from build123d import *

# Parameters (mm, degrees)
ESQUISSE1_R        = 10
ESQUISSE1_R_2      = 2.1
BOSS_EXTRU_1_DEPTH = 3
BOSS_EXTRU_2_DEPTH = 5
BOSS_EXTRU_3_START = 2.45
BOSS_EXTRU_3_DEPTH = 2.45
ESQUISSE4_R        = 10
ESQUISSE4_R_2      = 8
BOSS_EXTRU_4_DEPTH = 2
CONG_5_R           = 2
CONG_6_R           = 2
CONG_7_R           = 2
CONG_8_R           = 2
CONG_10_R          = 0.5
CHANFREIN1_SIZE    = 0.2


with BuildPart() as part:
    # Esquisse1 → Boss.-Extru.1 (new body)
    with BuildSketch(Plane(origin=(0, 0, 0), x_dir=(1, 0, 0), z_dir=(0, 1, 0))):
        with Locations(Location((0, 0, 0), (0, 0, 270))):
            Circle(ESQUISSE1_R)
        with Locations(Location((0, 0, 0), (0, 0, 270))):
            Circle(ESQUISSE1_R_2, mode=Mode.SUBTRACT)
    extrude(amount=BOSS_EXTRU_1_DEPTH)

    # Esquisse2 → Boss.-Extru.2 (add)
    with BuildSketch(Plane(origin=(0, 0, 0), x_dir=(1, 0, 0), z_dir=(0, 1, 0))):
        with BuildLine():
            Line((-9.901515036, -1.4), (-16, -1.4))
            ThreePointArc((-16, -1.4), (-17.4, 0), (-16, 1.4))
            Line((-16, 1.4), (-9.901515036, 1.4))
            ThreePointArc((-9.901515036, 1.4), (-8.501515036, 0), (-9.901515036, -1.4))
        make_face()
        with BuildLine():
            Line((9.901515036, -1.4), (16, -1.4))
            ThreePointArc((16, -1.4), (17.4, 0), (16, 1.4))
            Line((16, 1.4), (9.901515036, 1.4))
            ThreePointArc((9.901515036, 1.4), (8.501515036, 0), (9.901515036, -1.4))
        make_face()
    extrude(amount=BOSS_EXTRU_2_DEPTH)

    # Esquisse3 → Boss.-Extru.3 (add)
    with BuildSketch(Plane.XZ.offset(BOSS_EXTRU_3_START)):
        with BuildLine():
            Line((-10.05, -1.4), (-16, -1.4))
            ThreePointArc((-16, -1.4), (-17.4, 0), (-16, 1.4))
            Line((-16, 1.4), (-10.05, 1.4))
            ThreePointArc((-10.05, 1.4), (-8.65, 0), (-10.05, -1.4))
        make_face()
        with BuildLine():
            Line((10.05, -1.4), (16, -1.4))
            ThreePointArc((16, -1.4), (17.4, 0), (16, 1.4))
            Line((16, 1.4), (10.05, 1.4))
            ThreePointArc((10.05, 1.4), (8.65, 0), (10.05, -1.4))
        make_face()
    extrude(amount=-BOSS_EXTRU_3_DEPTH)

    # Esquisse4 → Boss.-Extru.4 (add)
    with BuildSketch(Plane(origin=(0, 3, 0), x_dir=(1, 0, 0), z_dir=(0, 1, 0))):
        Circle(ESQUISSE4_R)
        with Locations(Location((0, 0, 0), (0, 0, 270))):
            Circle(ESQUISSE4_R_2, mode=Mode.SUBTRACT)
    extrude(amount=BOSS_EXTRU_4_DEPTH)

    # Congé5
    # the kernel refuses this fillet: 2 mm, written as the material it adds along each edge
    with BuildSketch(Plane(origin=(9.901515036, 5, -1.4), x_dir=(1, 0, 0), z_dir=(0, -1, 0))) as cong_5_piece_1:
        with BuildLine():
            CenterArc((1.606742869, -2), CONG_5_R, 90, 73.540750372)
            ThreePointArc((-0.311300115, -1.433333333), (-0.129335377, -0.72238185), (0, 0))
            Line((0, 0), (1.606742869, 0))
        make_face()
    extrude(amount=5)

    # Congé6
    # the kernel refuses this fillet: 2 mm, written as the material it adds along each edge
    with BuildSketch(Plane(origin=(9.901515036, 0, 1.4), x_dir=(1, 0, 0), z_dir=(0, 1, 0))) as cong_6_piece_1:
        with BuildLine():
            CenterArc((1.606742869, -2), CONG_6_R, 90, 73.540750372)
            ThreePointArc((-0.311300115, -1.433333333), (-0.129335377, -0.72238185), (0, 0))
            Line((0, 0), (1.606742869, 0))
        make_face()
    extrude(amount=5)

    # Congé7
    # the kernel refuses this fillet: 2 mm, written as the material it adds along each edge
    with BuildSketch(Plane(origin=(-9.901515036, 5, -1.4), x_dir=(0.2122381850229741, 0, -0.9772179658695156), z_dir=(0, -1, 0))) as cong_7_piece_1:
        with BuildLine():
            CenterArc((1.613423741, -1.994614368), CONG_7_R, 94.20570169, 73.540750372)
            Line((-0.34101219, -1.570137998), (0, 0))
            ThreePointArc((0, 0), (0.733374428, -0.026928159), (1.466748856, 0))
        make_face()
    extrude(amount=5)

    # Congé8
    # the kernel refuses this fillet: 2 mm, written as the material it adds along each edge
    with BuildSketch(Plane(origin=(-9.901515036, 5, 1.4), x_dir=(0.21223818502297503, 0, 0.9772179658695155), z_dir=(0, -1, 0))) as cong_8_piece_1:
        with BuildLine():
            CenterArc((1.613423741, 1.994614368), CONG_8_R, 192.253547938, 73.540750372)
            Line((-0.34101219, 1.570137998), (0, 0))
            ThreePointArc((0, 0), (0.733374428, 0.026928159), (1.466748856, 0))
        make_face()
    extrude(amount=5)

    # Congé10
    cong_10_edges = [part.edges().sort_by_distance(p)[0] for p in [
        (-8.65, -2.45, 0),
        (-13.025, -2.45, 1.4),
        (-17.4, -2.45, 0),
        (-13.025, -2.45, -1.4),
        (8.65, -2.45, 0),
        (13.025, -2.45, -1.4),
        (17.4, -2.45, 0),
        (13.025, -2.45, 1.4),
    ]]
    fillet(cong_10_edges, radius=CONG_10_R)

    # Chanfrein1
    chanfrein1_edges = [part.edges().sort_by_distance(p)[0] for p in [
        (0, 5, -8),
    ]]
    chamfer(chanfrein1_edges, length=CHANFREIN1_SIZE)


solid = part.part
Geometry check sheet. Reference: the model listing, model coordinates, mm. A direction names the side the tool comes from. Give positions to 0.01 mm unless a question says otherwise; leave off trailing zeros. Order: outer loops, then holes, each group sorted by start corner. A loop starts at its lowest first (then second) coordinate and runs counter-clockwise, first axis right, second up.
1) Draft check along Z on faces 4 (the cylindrical face through (-7.81, 3.89, -1.73)), 5 (the cylindrical face through (-10.325, 2.535, 1.787)), 6 (the cylindrical face through (0, 2, -10)). Enter one of: released by +Z, released by -Z, zero draft, split by the parting line, or undercut.
Results are:
face 4: undercut
face 5: released by +Z
face 6: released by -Z
2) Tool access check on faces 1 (the flat face through (-2, 3, 2)), 2 (the cylindrical face through (17.4, 1.5, 0)), 3 (the cylindrical face through (8.65, -0.99, 0.03)). Record the directions out of +Z, -Z, +X, -X, +Y, -Y that give a thin tool (end or side, any length) a straight path to the whole face; none if there is none.
Results are:
face 1: +Y
face 2: +X, +Y, -Y
face 3: -Y
3) Cross-section at B-B (y = -0.5). Record the boundary of the cut face in (x, z), then the cut area to 3 significant figures.
Results are:
outline: (-16, -1.4) - (-10.05, -1.4) arc R1.4 ccw to (-10.05, 1.4) - (-16, 1.4) arc R1.4 ccw to start; (10.05, -1.4) - (16, -1.4) arc R1.4 ccw to (16, 1.4) - (10.05, 1.4) arc R1.4 ccw to start
area: 45.6 mm2
4) Cross-section at C-C (y = 2.5). Record the boundary of the cut face in (x, z).
Results are:
outline: (-16, -1.4) - (-11.51, -1.4) arc R2 cw to (-9.59, -2.83) arc R10 ccw to (9.59, -2.83) arc R2 cw to (11.51, -1.4) - (16, -1.4) arc R1.4 ccw to (16, 1.4) - (11.51, 1.4) arc R2 cw to (9.59, 2.83) arc R10 ccw to (-9.59, 2.83) arc R2 cw to (-11.51, 1.4) - (-16, 1.4) arc R1.4 ccw to start; hole circle Ø4.2 at (0, 0)
5) Cross-section at D-D (x = 15). Record the boundary of the cut face in (y, z), then the cut area to 3 significant figures.
Results are:
outline: (-2.45, -0.9) arc R0.5 ccw to (-1.95, -1.4) - (5, -1.4) - (5, 1.4) - (-1.95, 1.4) arc R0.5 ccw to (-2.45, 0.9) - close
area: 20.8 mm2
6) Gauge pin test, flat ends, axial feed: pin 1 (3 mm diameter, centred on x = -12.5, y = 1, fed in from -Z); pin 2 (6 mm diameter, centred on x = -4.5, z = -4.5, fed in from -Y); pin 3 (1.8 mm diameter, centred on x = 12.5, y = 2, fed in from +Z). Record the tip position at first contact, or that the pin passes through.
Results are:
pin 1: stops at z = -1.47
pin 2: stops at y = 0
pin 3: stops at z = 1.4
7) Material ranges on probe 1 along X at (y, z) = (2.1, 0); probe 2 along Z at (x, y) = (-3.5, 3.5); probe 3 along Y at (x, z) = (9, -3.5), recorded low to high.
Results are:
probe 1: x = -17.4 to -2.1, 2.1 to 17.4
probe 2: z = -9.37 to -7.19, 7.19 to 9.37
probe 3: y = 0 to 5
8) Cross-section at A-A (z = 0). Record the boundary of the cut face in (x, y), then the cut area to 3 significant figures.
Results are:
outline: (-17.4, -1.95) arc R0.5 ccw to (-16.9, -2.45) - (-9.15, -2.45) arc R0.5 ccw to (-8.65, -1.95) - (-8.65, 0) - (-2.1, 0) - (-2.1, 3) - (-8, 3) - (-8, 4.8) - (-8.2, 5) - (-17.4, 5) - close; (2.1, 0) - (8.65, 0) - (8.65, -1.95) arc R0.5 ccw to (9.15, -2.45) - (16.9, -2.45) arc R0.5 ccw to (17.4, -1.95) - (17.4, 5) - (8.2, 5) - (8, 4.8) - (8, 3) - (2.1, 3) - close
area: 172 mm2
